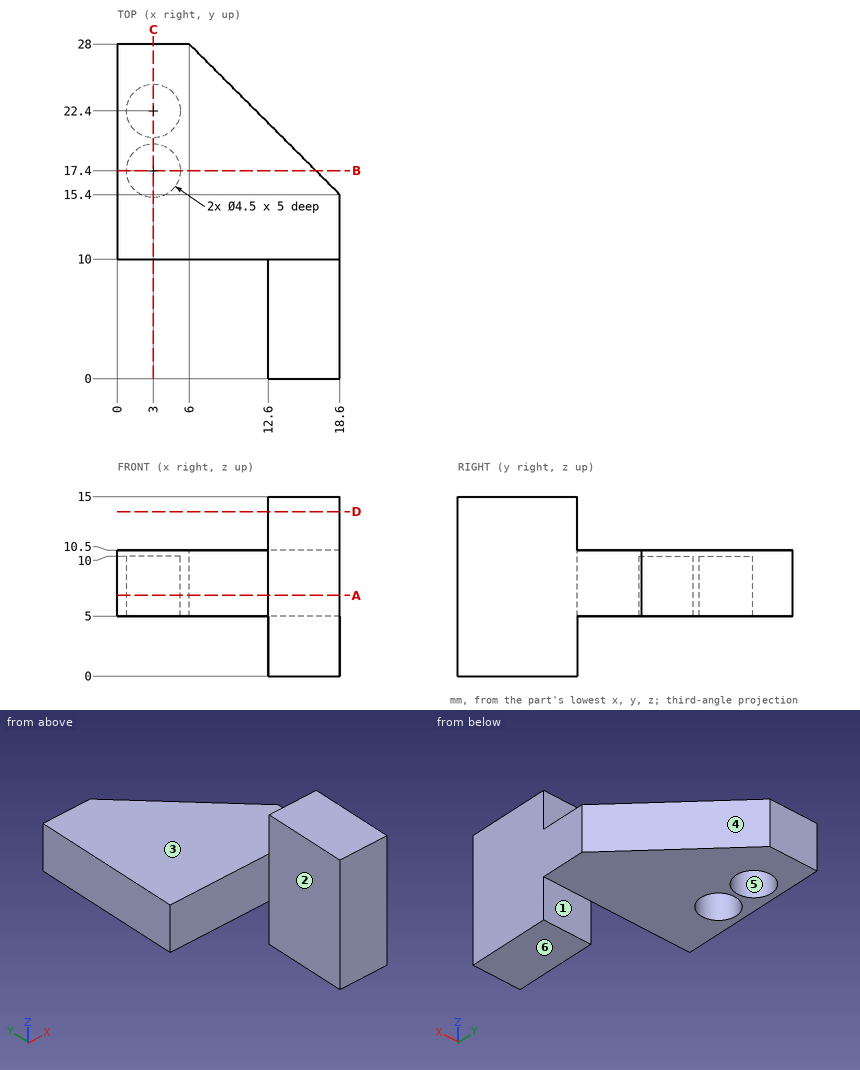
Verification items for this drawing (mm, ordinates from the low corner). A direction names the side the tool comes from. Coordinates: 2 decimals unless noted, no trailing zeros. Order: outer loops, then holes, each group sorted by start corner. A loop starts at its lowest first (then second) coordinate and runs counter-clockwise, first axis right, second up. Notation, with made-up numbers: M 88,-2.5 L 98,-2.5 A32 ccw 98,35.5 Z; hole C 6.25,39 d5. An arc over 180 degrees is marked long. One line per item, written item: value. Start each with the question number.
Item 1: Access from +Z, -Z, +X, -X, +Y, -Y to the whole of each face (thin tool, end or side, straight path). Record for the marked faces 1, 2 and 3.
Item 2: Thickness scan on probe 1 along Y at (x, z) = (3, 8.1); probe 2 along Y at (x, z) = (18.25, 4.25); probe 3 along Z at (x, y) = (10.5, 14.5). Record the ranges inside material, lowest first.
Item 3: Sectioned sample at D-D on z = 13.75. Record the cut outline in (x, y).
Item 4: Sectioned sample at C-C on x = 3. Record the cut outline in (y, z), then the cut area to 3 significant figures.
Item 5: Mould release check, pull along X, two halves, no side actions. Record for the marked faces 4, 5 and 6: pulls with the +X half, pulls with the -X half, needs draft (parallel to the pull), parting line crosses it, or undercut.
Item 6: Sectioned sample at A-A on z = 6.75. Record the cut outline in (x, y), then the cut area to 3 significant figures.
Item 7: Depth check by flat-ended pin: P1, Ø2.5, axis at x = 16.5, z = 2.5, coming from the +Y side; P2, Ø9, axis at x = 7.5, y = 20, coming from the -Z side; P3, Ø3.5, axis at x = 3, y = 22.4, coming from the +Z side; P4, Ø1.5, axis at x = 15, y = 21.5, coming from the -Z side. Enter the tip coordinate at first touch or a pass-through.
Item 8: Sectioned sample at B-B on y = 17.4. Record the cut outline in (x, z), then the cut area to 3 significant figures.
Calculated:
1. face 1: -Z, +X, -X, +Y
1. face 2: +Z, -Z, -X, -Y
1. face 3: +Z, +X, -X, +Y
2. probe 1: 10 to 15.15, 19.65 to 20.15, 24.65 to 28
2. probe 2: 0 to 10
2. probe 3: 5 to 10.5
3. outline: M 12.6,0 L 18.6,0 L 18.6,10 L 12.6,10 Z
4. outline: M 10,5 L 15.15,5 L 15.15,10 L 19.65,10 L 19.65,5 L 20.15,5 L 20.15,10 L 24.65,10 L 24.65,5 L 28,5 L 28,10.5 L 10,10.5 Z
4. area: 54.0 mm^2
5. face 4: pulls with the +X half
5. face 5: undercut
5. face 6: needs draft
6. outline: M 0,10 L 12.6,10 L 12.6,0 L 18.6,0 L 18.6,15.4 L 6,28 L 0,28 Z; hole C 3,17.4 d4.5; hole C 3,22.4 d4.5
6. area: 284 mm^2
7. P1: y = 10
7. P2: z = 5
7. P3: z = 10.5
7. P4: through
8. outline: M 0,5 L 0.75,5 L 0.75,10 L 5.25,10 L 5.25,5 L 16.6,5 L 16.6,10.5 L 0,10.5 Z
8. area: 68.8 mm^2
